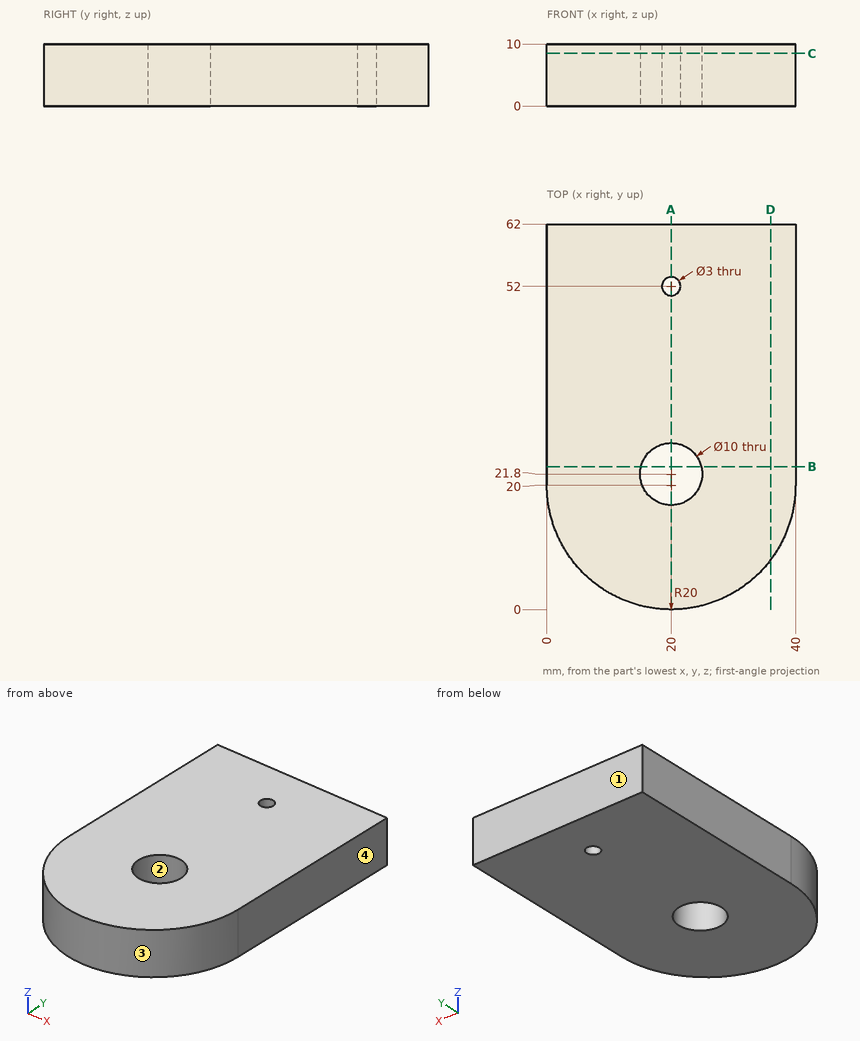
The figure shows three views and two pictorial views of one solid part (mm, origin at its lowest corner). Answer the questions. Give positions to 0.01 mm unless a question says otherwise; leave off trailing zeros. Write each loop counter-clockwise with the first axis right and the second up, starting at its lowest first coordinate (ties: lowest second). Pieces come first, ordered by that corner, then holes. Notation, with made-up numbers: (-14.75, 10.25) -> (17.25, 10.25) arc R22 ccw to (17.25, 45.25) -> close; hole circle Ø9 at (75, -4.75). An arc over 180 degrees is marked (long way). Write each question's results on one line, items separated by ' | '.
1. Find section B-B on y = 23. Determine the outline of the cut face in (x, z).
Data:
outline: (0, 0) -> (15.15, 0) -> (15.15, 10) -> (0, 10) -> close; (24.85, 0) -> (40, 0) -> (40, 10) -> (24.85, 10) -> close
2. Find section A-A on x = 20. Determine the outline of the cut face in (y, z).
Data:
outline: (0, 0) -> (16.8, 0) -> (16.8, 10) -> (0, 10) -> close; (26.8, 0) -> (50.5, 0) -> (50.5, 10) -> (26.8, 10) -> close; (53.5, 0) -> (62, 0) -> (62, 10) -> (53.5, 10) -> close
3. Find section D-D on x = 36. Determine the outline of the cut face in (y, z), and give its area (3 significant figures).
Data:
outline: (8, 0) -> (62, 0) -> (62, 10) -> (8, 10) -> close | area: 540 mm^2
4. Determine the mould class of the marked faces 1, 2, 3 and 4 for opening direction Y: +Y half, -Y half, draft (parallel to the pull), parting line (faces both ways), or undercut.
Data:
face 1: +Y half | face 2: undercut | face 3: -Y half | face 4: draft
5. Straight lines are drawn through the part: L1, parallel to Y at x = 20, z = 2.75; L2, parallel to X at y = 52, z = 6.75; L3, parallel to Y at x = 23, z = 5.25. For each, find the intervals that lie inside material, in ascending order.
Data:
L1: 0 to 16.8, 26.8 to 50.5, 53.5 to 62 | L2: 0 to 18.5, 21.5 to 40 | L3: 0.23 to 17.8, 25.8 to 62
6. Find section C-C on z = 8.5. Determine the outline of the cut face in (x, y), and give its area (3 significant figures).
Data:
outline: (0, 20) arc R20 ccw to (40, 20) -> (40, 62) -> (0, 62) -> close; hole circle Ø10 at (20, 21.8); hole circle Ø3 at (20, 52) | area: 2,220 mm^2
7. This flat-tipped pin is pushed along its axis until it touches: pin 1 Ø8 at (x, y) = (20, 21.8) entering from +Z. Where does it stop, or does it pass through?
Data:
pin 1: through
